from build123d import *

# Parameters (mm, degrees)
F0_W     = 120.2
F0_H     = 97
F0_W_2   = 2.5
F0_H_2   = 0.03408
F1_DEPTH = 5.9
F0_H_3   = 120.46592
F2_DEPTH = 6.9
F3_DEPTH = 1.2


with BuildPart() as f1:
    # F0 (on Front) → F1 (new body)
    with BuildSketch(Plane.XZ):
        Polygon((51.5, 60.25), (-86.5, 60.25), (-86.5, -60.25), (86.5, -60.25), (86.5, 60.25), (54, 60.25), (54, -60.21592), (51.5, -60.21592), align=None)
        with Locations((-10.6, 0)):
            Rectangle(F0_W, F0_H, mode=Mode.SUBTRACT)
        with Locations((52.75, 60.26704)):
            Rectangle(F0_W_2, F0_H_2)
    extrude(amount=F1_DEPTH)

    # F0 (on Front) → F2 (join)
    with BuildSketch(Plane.XZ):
        with Locations((52.75, 0.01704)):
            Rectangle(F0_W_2, F0_H_3)
    extrude(amount=F2_DEPTH)

    # F0 (on Front) → F3 (join)
    with BuildSketch(Plane.XZ):
        with Locations((-10.6, 0)):
            Rectangle(F0_W, F0_H)
    extrude(amount=F3_DEPTH)

    # F4: F1 across face


with BuildPart() as f1_1:
    add(f1.part)
    add(f1.part.mirror(Plane(origin=(0.000216, 0, 0.000246), x_dir=(1, 0, 0), z_dir=(0, 1, 0))))


solid = f1_1.part
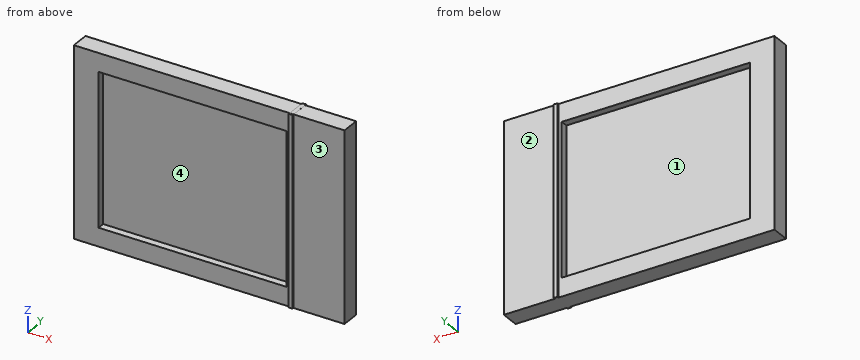
Verification items for the finished model (mm, model axes). Face numbers are marked on the shaded views. A direction names the side the tool comes from. Round coordinates to 2 decimals unless told otherwise and drop trailing zeros. Order: outer loops, then holes, each group sorted by start corner. A loop starts at its lowest first (then second) coordinate and runs counter-clockwise, first axis right, second up. Notation, with made-up numbers: (-9.75, 60) -> (7.25, 60) arc R24 ccw to (7.25, 89) -> close; hole circle Ø6 at (86, -15). An arc over 180 degrees is marked (long way). Put each result on its own line as item: value.
1) Mould release check, pull along X, two halves, no side actions. Record for the marked faces 1 and 2: +X half, -X half, draft (parallel to the pull), parting line (faces both ways), or undercut.
Final values:
face 1: undercut
face 2: draft
2) Set-up check for the marked faces 3 and 4: record each of +Z, -Z, +X, -X, +Y, -Y from which the full face is reachable in a straight line by a thin tool's end or side.
Final values:
face 3: +Z, -Z, -Y
face 4: -Y
3) Material ranges on line 1 (Z direction, x = -38, y = -5.75); line 2 (X direction, y = 2, z = -22); line 3 (Z direction, x = 74.5, y = 3.75), recorded low to high.
Final values:
line 1: z = -60.25 to -48.5, 48.5 to 60.25
line 2: x = -86.5 to -70.7, 49.5 to 86.5
line 3: z = -60.25 to 60.25
4) Section check B-B (x = 26.5). Record the cut outline in (y, z).
Final values:
outline: (-5.9, -60.25) -> (5.9, -60.25) -> (5.9, -48.5) -> (1.2, -48.5) -> (1.2, 48.5) -> (5.9, 48.5) -> (5.9, 60.25) -> (-5.9, 60.25) -> (-5.9, 48.5) -> (-1.2, 48.5) -> (-1.2, -48.5) -> (-5.9, -48.5) -> close
5) Section check D-D (z = 50.5). Record the cut outline in (x, y), then the cut area to 3 significant figures.
Final values:
outline: (-86.5, -5.9) -> (51.5, -5.9) -> (51.5, -6.9) -> (54, -6.9) -> (54, -5.9) -> (86.5, -5.9) -> (86.5, 5.9) -> (54, 5.9) -> (54, 6.9) -> (51.5, 6.9) -> (51.5, 5.9) -> (-86.5, 5.9) -> close
area: 2,050 mm^2
6) Depth check by flat-ended pin: pin 1 (1.1 mm diameter, centred on y = -6.5, z = -5.5, fed in from +X); pin 2 (10 mm diameter, centred on x = -10, z = -12, fed in from -Y); pin 3 (1.4 mm diameter, centred on x = -28.5, y = -4, fed in from +Z). Enter the tip coordinate at first touch or a pass-through.
Final values:
pin 1: stops at x = 54
pin 2: stops at y = -1.2
pin 3: stops at z = 60.25
7) Section check C-C (z = 0). Record the cut outline in (x, y).
Final values:
outline: (-86.5, -5.9) -> (-70.7, -5.9) -> (-70.7, -1.2) -> (49.5, -1.2) -> (49.5, -5.9) -> (51.5, -5.9) -> (51.5, -6.9) -> (54, -6.9) -> (54, -5.9) -> (86.5, -5.9) -> (86.5, 5.9) -> (54, 5.9) -> (54, 6.9) -> (51.5, 6.9) -> (51.5, 5.9) -> (49.5, 5.9) -> (49.5, 1.2) -> (-70.7, 1.2) -> (-70.7, 5.9) -> (-86.5, 5.9) -> close
